Input: dimensioned drawing with shaded views. Units: mm. Origin: part minimum x, y, z. Coordinates: 2 decimals unless noted, no trailing zeros. Write each loop counter-clockwise with the first axis right and the second up, starting at its lowest first coordinate (ties: lowest second). Pieces come first, ordered by that corner, then holes. Notation, with made-up numbers: (-14.75, -3.75) -> (-10.75, -3.75) arc R10 cw to (-10.75, 8.25) -> close; hole circle Ø8 at (10, -6.75). An arc over 180 degrees is marked (long way). One line per item, written item: value. Start each with the question number.
1. Section query C-C, the plane x = 54.25. Output: boundary loops of the cut face in (y, z), and give its area (3 significant figures).
2. Section query A-A, the plane z = 33.5. Output: boundary loops of the cut face in (x, y).
3. Section query B-B, the plane x = 36. Output: boundary loops of the cut face in (y, z), and give its area (3 significant figures).
4. Line query: line 1 (X direction, y = 7, z = 33.5); line 2 (Z direction, x = 34, y = 9) (1 decimal). Output: solid intervals per line, ascending.
5. First-contact query: P1, Ø6, axis at x = 27.5, y = 5.5, coming from the -Z side. Flat tip, straight axial feed; report the tip coordinate or a pass-through.
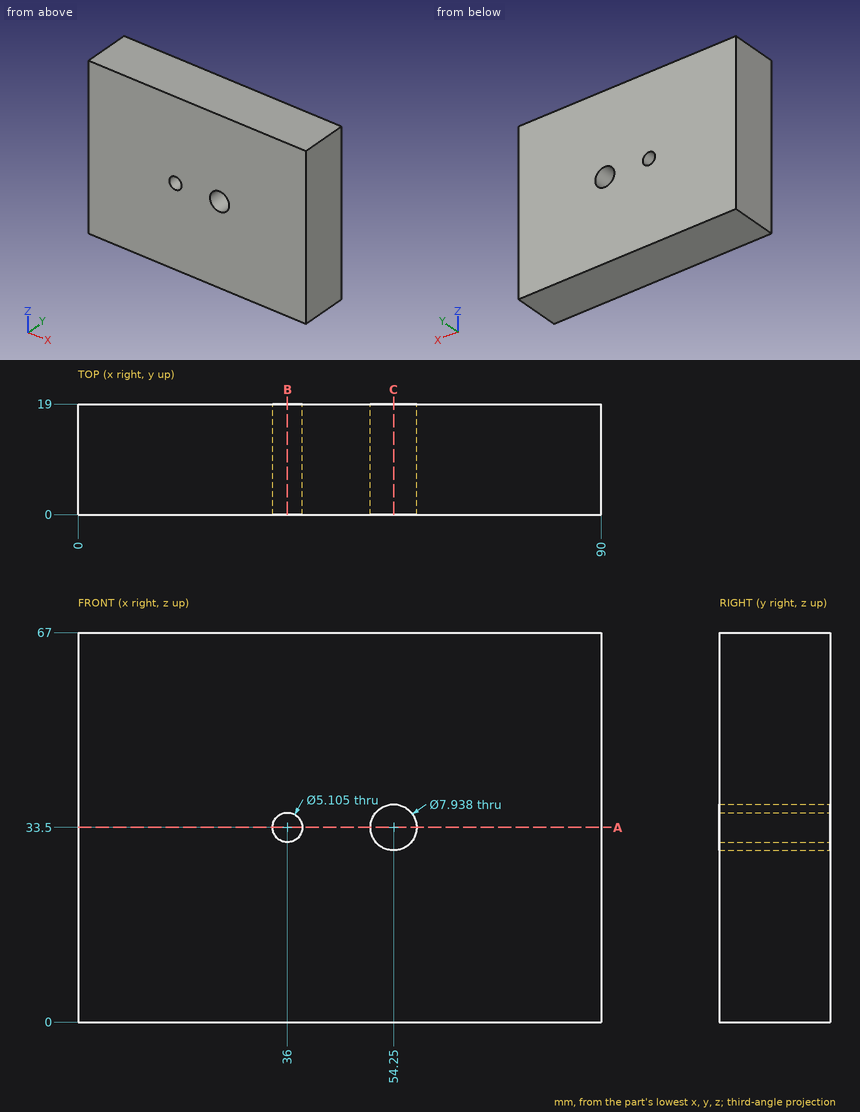
Computed values:
1. outline: (0, 0) -> (19, 0) -> (19, 29.53) -> (0, 29.53) -> close; (0, 37.47) -> (19, 37.47) -> (19, 67) -> (0, 67) -> close
1. area: 1,120 mm²
2. outline: (0, 0) -> (33.45, 0) -> (33.45, 19) -> (0, 19) -> close; (38.55, 0) -> (50.28, 0) -> (50.28, 19) -> (38.55, 19) -> close; (58.22, 0) -> (90, 0) -> (90, 19) -> (58.22, 19) -> close
3. outline: (0, 0) -> (19, 0) -> (19, 30.95) -> (0, 30.95) -> close; (0, 36.05) -> (19, 36.05) -> (19, 67) -> (0, 67) -> close
3. area: 1,180 mm²
4. line 1: x = 0 to 33.45, 38.55 to 50.28, 58.22 to 90
4. line 2: z = 0 to 31.9, 35.1 to 67
5. P1: stops at z = 0
